Source: CAD feature listing. Evaluate the final solid. Frame: model axes, mm. A direction names the side the tool comes from. Give positions to 0.01 mm unless a question says otherwise; leave off trailing zeros. Order: outer loops, then holes, each group sorted by start corner. A loop starts at its lowest first (then second) coordinate and runs counter-clockwise, first axis right, second up. Notation, with made-up numbers: M 81,9.25 L 113,9.25 A24 ccw 113,48.25 Z; hole C -5.5,11 d9. An arc over 180 degrees is marked long. Use CSV: the item, a comma, the result in double quotes. Start each with the question number.
Item 1: Section query D-D on y = 160.5. Return loops of the section in (x, z).
Item 2: Ray query, probe 1 along X at (y, z) = (27, 9); probe 2 along Z at (x, y) = (-77.5, 218.5); probe 3 along Y at (x, z) = (1, 107.5). Return the intervals inside material, ascending. Write a range as from..to.
Item 3: First-contact query: pin 1 (1 mm diameter, centred on x = -9.5, y = -170.5, fed in from +Z); pin 2 (8 mm diameter, centred on x = 32, z = 25, fed in from +Y); pin 3 (9.5 mm diameter, centred on x = -9.5, z = 18.5, fed in from +Y). Flat tips, straight axial feed; report the tip coordinate or a pass-through.
Item 4: Section query B-B on x = 0. Return loops of the section in (y, z).
Item 5: Access query for faces 4 (the face through (16.5, 44, 8)), 5 (the face through (29.4, -56, 54)), 6 (the face through (0, -95.173, 65)), 7 (the face through (-29.4, -56, 54)). Directions: +Z, -Z, +X, -X, +Y, -Y. A direction counts if a zero-diameter tool reaches every point of the face in a straight line with its end or side. Return the directions, or none.
Item 6: Pull-direction query (X, two-part tool) for faces 1 (the face through (134.964, -235.742, 7.395)), 2 (the face through (0, 15, 8)), 3 (the face through (0, 7.107, 21)); classes: +X half, -X half, draft (parallel to the pull), parting line (faces both ways), or undercut.
Item 7: Section query C-C on z = 70.5. Return loops of the section in (x, y).
Item 8: Section query A-A on y = 65.5. Return loops of the section in (x, z), and give its area (4 significant figures).
from build123d import *

# Parameters (mm, degrees)
F1_DEPTH = 15
F2_W     = 33
F2_H     = 58
F3_DEPTH = 15.001
F4_W     = 58.8
F4_H     = 102.2799882368
F5_DEPTH = 101.6
F6_SIZE  = 70
F7_SIZE  = 20


with BuildPart() as f1:
    # F0 (on Top) → F1 (new body)
    with BuildSketch(Plane.XY):
        with BuildLine():
            Line((-100, -250), (100, -250))
            ThreePointArc((100, -250), (135.3553390593, -235.3553390593), (150, -200))
            Line((150, -200), (150, 100))
            ThreePointArc((150, 100), (0, 250), (-150, 100))
            Line((-150, 100), (-150, -200))
            ThreePointArc((-150, -200), (-135.3553390593, -235.3553390593), (-100, -250))
        make_face()
    extrude(amount=F1_DEPTH)

    # F2 (on face) → F3 (cut, through all)
    with BuildSketch(Plane.XY.offset(15)):
        with Locations((0, 44)):
            Rectangle(F2_W, F2_H)
    extrude(amount=-F3_DEPTH, mode=Mode.SUBTRACT)

    # F4 (on face) → F5 (join)
    with BuildSketch(Plane.XY.offset(15)):
        with Locations((0, -44.0329860869)):
            Rectangle(F4_W, F4_H)
    extrude(amount=F5_DEPTH)

    # F6
    f6_edges = [f1.edges().sort_by_distance(p)[0] for p in [
        (0, 7.107008, 116.6),
    ]]
    chamfer(f6_edges, length=F6_SIZE)

    # F7
    f7_edges = [f1.edges().sort_by_distance(p)[0] for p in [
        (0, 7.107008, 46.6),
    ]]
    chamfer(f7_edges, length=F7_SIZE)


solid = f1.part
Verdict:
1,outline,"M -137.26,0 L 137.26,0 L 137.26,15 L -137.26,15 Z"
2,probe 1,"-150..-16.5, 16.5..150"
2,probe 2,"0..15"
2,probe 3,"-95.17..-53.79"
3,pin 1,"z = 15"
3,pin 2,"y = 7.11"
3,pin 3,"y = 249.87"
4,outline,"M -250,0 L 15,0 L 15,15 L 7.11,15 L 7.11,26.6 L -7.04,60.74 L -62.89,116.6 L -95.17,116.6 L -95.17,15 L -250,15 Z; M 73,0 L 250,0 L 250,15 L 73,15 Z"
5,face 4,"+Z, -Z"
5,face 5,"+Z, +X, +Y, -Y"
5,face 6,"+Z, +X, -X, -Y"
5,face 7,"+Z, -X, +Y, -Y"
6,face 1,"+X half"
6,face 2,"undercut"
6,face 3,"draft"
7,outline,"M -29.4,-95.17 L 29.4,-95.17 L 29.4,-16.79 L -29.4,-16.79 Z"
8,outline,"M -150,0 L -16.5,0 L -16.5,15 L -150,15 Z; M 16.5,0 L 150,0 L 150,15 L 16.5,15 Z"
8,area,"4,005 mm2"
